For this review, take the finished solid that the model builds, in its own axes (mm). Coordinates: 2 decimals unless noted, no trailing zeros. Write each loop counter-clockwise with the first axis right and the second up, starting at its lowest first coordinate (ties: lowest second). Pieces come first, ordered by that corner, then holes. Notation, with made-up numbers: (-38, 30.25) - (8, 30.25) arc R13 ccw to (8, 35.25) - close; hole circle Ø2 at (66, -0.75). An arc over 180 degrees is marked (long way). Write each question's results on one line, items separated by ' | '.
from build123d import *

# Parameters (mm, degrees)
SKETCH_1_W            = 9
SKETCH_1_H            = 50
EXTRUDE_1_DEPTH       = 2
HOLE_WIZARD_M41_D     = 3.3
HOLE_WIZARD_M41_DEPTH = 11.5
HOLE_WIZARD_M41_TIP   = 0.991420021
FILLET_1_R            = 2


with BuildPart() as part:
    # Эскиз1 → Бобышка-Вытянуть1 (new body)
    with BuildSketch(Plane.XY):
        Rectangle(SKETCH_1_W, SKETCH_1_H)
    extrude(amount=EXTRUDE_1_DEPTH)

    # Отверстие обработанное метчиком M41
    with Locations(Plane.XY.offset(2)):
        with Locations((0, -10), (0, 20), (0, 10), (0, -20)):
            Hole(HOLE_WIZARD_M41_D / 2, depth=HOLE_WIZARD_M41_DEPTH)
            with Locations((0, 0, -(HOLE_WIZARD_M41_DEPTH + HOLE_WIZARD_M41_TIP / 2))):  # 118° drill point
                Cone(0, HOLE_WIZARD_M41_D / 2, HOLE_WIZARD_M41_TIP, mode=Mode.SUBTRACT)

    # Скругление1
    fillet_1_edges = [part.edges().sort_by_distance(p)[0] for p in [
        (4.5, -25, 1),
        (-4.5, -25, 1),
        (-4.5, 25, 1),
        (4.5, 25, 1),
    ]]
    fillet(fillet_1_edges, radius=FILLET_1_R)


solid = part.part
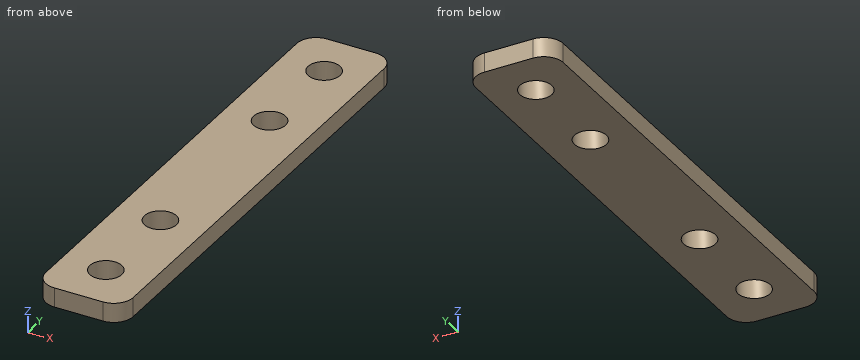
Q1. Wall thickness on line 1 along Y through (x, z) = (0, 0.85); line 2 along Y through (x, z) = (1.5, 1.5); line 3 along X through (y, z) = (21.5, 0.15): over which ranges is each line inside the solid? List them lowest first. Write a range as from..to.
Results found:
line 1: -25..-21.65, -18.35..-11.65, -8.35..8.35, 11.65..18.35, 21.65..25 | line 2: -25..-20.69, -19.31..-10.69, -9.31..9.31, 10.69..19.31, 20.69..25 | line 3: -4.5..-0.69, 0.69..4.5
Q2. Take a section at C-C on y = -20. State the section outline as (x, z) points.
Results found:
outline: (-4.5, 0) - (-1.65, 0) - (-1.65, 2) - (-4.5, 2) - close; (1.65, 0) - (4.5, 0) - (4.5, 2) - (1.65, 2) - close
Q3. Take a section at B-B on z = 1.65. State the section outline as (x, y) points.
Results found:
outline: (-4.5, -23) arc R2 ccw to (-2.5, -25) - (2.5, -25) arc R2 ccw to (4.5, -23) - (4.5, 23) arc R2 ccw to (2.5, 25) - (-2.5, 25) arc R2 ccw to (-4.5, 23) - close; hole circle Ø3.3 at (0, -20); hole circle Ø3.3 at (0, -10); hole circle Ø3.3 at (0, 10); hole circle Ø3.3 at (0, 20)
Q4. For pin 1 (3 mm diameter, centred on x = 0, y = 20, fed in from +Z), flat-tipped, find the tip position at first contact; note if it passes through.
Results found:
pin 1: through
Q5. Take a section at A-A on x = 0. State the section outline as (y, z) points.
Results found:
outline: (-25, 0) - (-21.65, 0) - (-21.65, 2) - (-25, 2) - close; (-18.35, 0) - (-11.65, 0) - (-11.65, 2) - (-18.35, 2) - close; (-8.35, 0) - (8.35, 0) - (8.35, 2) - (-8.35, 2) - close; (11.65, 0) - (18.35, 0) - (18.35, 2) - (11.65, 2) - close; (21.65, 0) - (25, 0) - (25, 2) - (21.65, 2) - close
